For this review, use the dimensioned drawing (mm, ordinates from the lowest corner) and the shaded views. Coordinates: 2 decimals unless noted, no trailing zeros. Loops run counter-clockwise (first coordinate to the right, second up) from the corner with the lowest first, then second, coordinate; pieces in that order, holes last. Notation, with made-up numbers: M 32.5,64 L 82.5,64 A14 cw 82.5,84 Z; hole C 39,88 d1. An arc over 180 degrees is marked long. One line per item, written item: value.
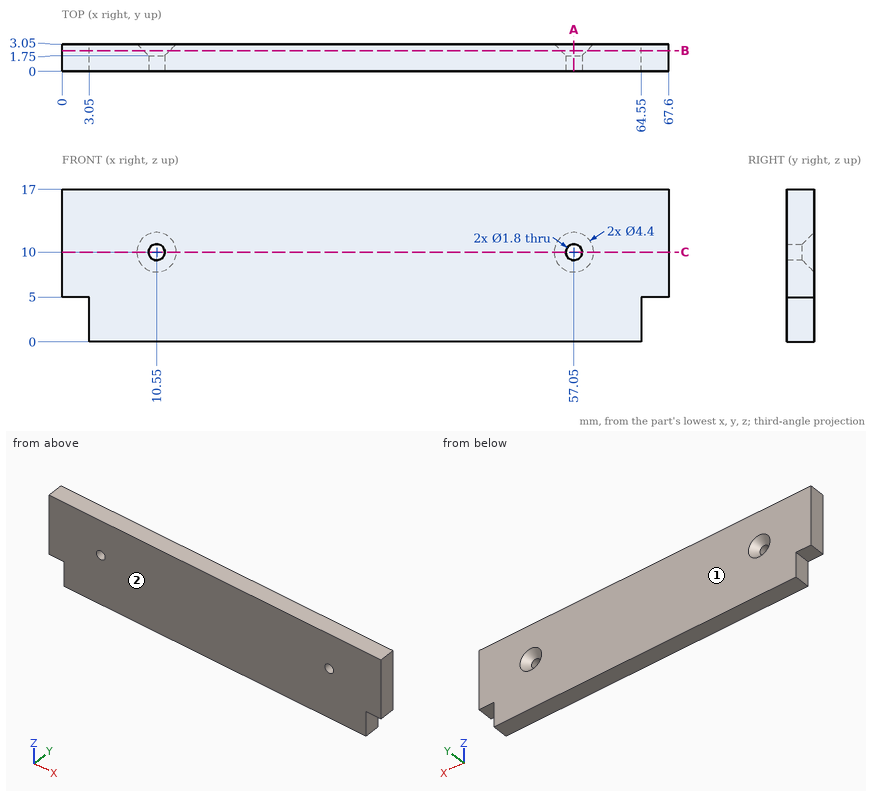
(1) To check wall thickness, follow line 1 along X through (y, z) = (0.8, 10); line 2 along Z through (x, y) = (10.55, 1.3); line 3 along X through (y, z) = (0.95, 1.75). State the ranges of each line that lie inside material, in increasing order. Write a range as [from, to].
Reply:
line 1: x = [0, 9.65], [11.45, 56.15], [57.95, 67.6]
line 2: z = [0, 9.1], [10.9, 17]
line 3: x = [3.05, 64.55]
(2) We need section B-B on y = 2.3. State the section outline as (x, z) points.
Reply:
outline: M 0,5 L 3.05,5 L 3.05,0 L 64.55,0 L 64.55,5 L 67.6,5 L 67.6,17 L 0,17 Z; hole C 10.55,10 d2.9; hole C 57.05,10 d2.9
(3) We need section A-A on x = 57.05. State the section outline as (y, z) points, then the cut area to 3 significant figures.
Reply:
outline: M 0,0 L 3.05,0 L 3.05,7.8 L 1.75,9.1 L 0,9.1 Z; M 0,10.9 L 1.75,10.9 L 3.05,12.2 L 3.05,17 L 0,17 Z
area: 44.7 mm2
(4) We need section C-C on z = 10. State the section outline as (x, y) points, then the cut area to 3 significant figures.
Reply:
outline: M 0,0 L 9.65,0 L 9.65,1.75 L 8.35,3.05 L 0,3.05 Z; M 11.45,0 L 56.15,0 L 56.15,1.75 L 54.85,3.05 L 12.75,3.05 L 11.45,1.75 Z; M 57.95,0 L 67.6,0 L 67.6,3.05 L 59.25,3.05 L 57.95,1.75 Z
area: 192 mm2
(5) Insertion check: pin 1 (3 mm diameter, centred on x = 10.55, z = 10, fed in from -Y); pin 2 (1.5 mm diameter, centred on y = 1, z = 3, fed in from -X); pin 3 (0.9 mm diameter, centred on y = 2, z = 3.5, fed in from +X); pin 4 (1.5 mm diameter, centred on x = 66, y = 1, fed in from -Z). Each pin has a flat end and moves straight along its axis. Give the tip position at first contact, or say it passes through.
Reply:
pin 1: stops at y = 0
pin 2: stops at x = 3.05
pin 3: stops at x = 64.55
pin 4: stops at z = 5
(6) Mouldability with a two-part tool opening along Y and no side actions: class the marked faces 1 and 2 as released by +Y, released by -Y, zero draft, split by the parting line, or undercut.
Reply:
face 1: released by +Y
face 2: released by -Y
